Part print with two shaded views. Sizes in mm from the minimum x, y, z corner. A direction names the side the tool comes from. Give positions to 0.01 mm unless a question says otherwise; leave off trailing zeros. Write each loop counter-clockwise with the first axis right and the second up, starting at its lowest first coordinate (ties: lowest second). Pieces come first, ordered by that corner, then holes. Notation, with made-up numbers: (82.25, 52) - (88.25, 52) arc R17 ccw to (88.25, 75) - close; hole circle Ø7 at (11, 28). An arc over 180 degrees is marked (long way). Answer as a JSON object with one key per item and string values.
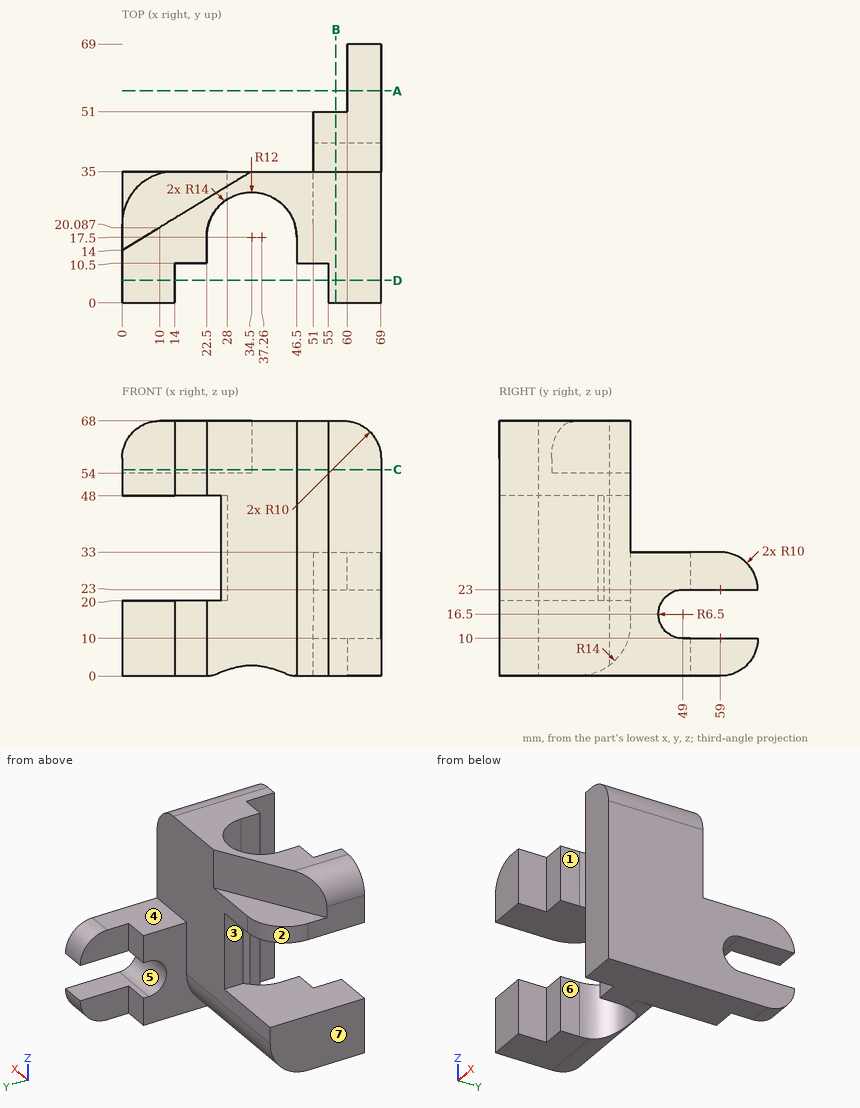
(1) Flat gauge pins, fed straight in: P1, Ø2, axis at x = 58.5, z = 29, coming from the +Y side; P2, Ø2, axis at x = 36.5, y = 36.5, coming from the -Z side; P3, Ø9, axis at x = 62.5, y = 42.5, coming from the +Z side; P4, Ø7.5, axis at y = 30.5, z = 37, coming from the -X side. Where does each tip first touch, or does it go through?
Answer key:
{"P1": "stops at y = 51", "P2": "passes through", "P3": "stops at z = 33", "P4": "stops at x = 26.75"}
(2) Saw through at A-A, the plane y = 56.5. Give the cut face in (x, z).
Answer key:
{"outline": "(60, 0) - (69, 0) - (69, 10) - (60, 10) - close; (60, 23) - (69, 23) - (69, 33) - (60, 33) - close"}
(3) Saw through at D-D, the plane y = 6. Give the cut face in (x, z), and give its area (3 significant figures).
Answer key:
{"outline": "(0, 0) - (14, 0) - (14, 20) - (0, 20) - close; (0, 48) - (14, 48) - (14, 68) - (10, 68) arc R10 ccw to (0, 58) - close; (55, 0) - (69, 0) - (69, 58) arc R10 ccw to (59, 68) - (55, 68) - close", "area": "1,470 mm²"}
(4) Saw through at C-C, the plane z = 55. Give the cut face in (x, y).
Answer key:
{"outline": "(0, 0) - (14, 0) - (14, 10.5) - (22.5, 10.5) - (22.5, 17.5) arc R12 cw to (46.5, 17.5) - (46.5, 10.5) - (55, 10.5) - (55, 0) - (69, 0) - (69, 35) - (34.5, 35) - (0, 14) - close"}
(5) 3-axis set-ups, long thin cutter, end or side, ignore diameter. For the marked faces 1, 2, 3 and 4: which of +Z, -Z, +X, -X, +Y, -Y reach the whole face in a straight line?
Answer key:
{"face 1": "+Z, -Z, -Y", "face 2": "+Z, -X, +Y", "face 3": "-X, +Y", "face 4": "+Z, +X, -X, +Y"}
(6) Pull direction X, two halves, no side cores. Call the marked faces 5, 6 and 7: pulls with the +X half, pulls with the -X half, needs draft (parallel to the pull), parting line crosses it, or undercut.
Answer key:
{"face 5": "needs draft", "face 6": "undercut", "face 7": "pulls with the -X half"}
(7) Saw through at B-B, the plane x = 57. Give the cut face in (y, z), and give its area (3 significant figures).
Answer key:
{"outline": "(0, 0) - (51, 0) - (51, 10) - (49, 10) arc R6.5 cw to (49, 23) - (51, 23) - (51, 33) - (35, 33) - (35, 68) - (0, 68) - close", "area": "2,820 mm²"}
(8) Probe L1, parallel to Y at x = 54, z = 27.5; L2, parallel to X at y = 11, z = 19.5; L3, parallel to Y at x = 50, z = 17. List the from-to ranges inside material, lowest first. Write a range as [from, to].
Answer key:
{"L1": "y = [10.5, 51]", "L2": "x = [0, 22.5], [46.5, 69]", "L3": "y = [10.5, 35]"}
